Source: CAD feature listing. Evaluate the final solid. Frame: model axes, mm. A direction names the side the tool comes from. Give positions to 0.01 mm unless a question says otherwise; leave off trailing zeros. Loops run counter-clockwise (first coordinate to the right, second up) from the corner with the lowest first, then second, coordinate; pieces in that order, holes last. Notation, with made-up numbers: (9, 16.25) - (47, 16.25) arc R14 cw to (47, 20.25) - close; hole circle Ø5 at (89, 67). An arc over 180 degrees is marked (long way). Put each result on its own line as item: value.
```python
from build123d import *

# Parameters (mm, degrees)
F1_DEPTH  = 6.35
F0_W      = 7.9375
F0_H      = 7.9375
F2_DEPTH  = 12.7
F3_DEPTH  = 127
F5_DEPTH  = 50.8
F6_W      = 7.9502
F6_H      = 7.9502
F7_DEPTH  = 113.03
F8_W      = 44.45
F8_H      = 3.175
F9_DEPTH  = 6.35
F10_W     = 50.8
F10_H     = 3.175
F11_DEPTH = 3.175


with BuildPart() as f1:
    # F0 (on Top) → F1 (new body)
    with BuildSketch(Plane.XY):
        with BuildLine():
            ThreePointArc((-100.0125, -39.6875), (-96.292756, -48.667756), (-87.3125, -52.3875))
            Line((-87.3125, -52.3875), (87.3125, -52.3875))
            ThreePointArc((87.3125, -52.3875), (96.292756, -48.667756), (100.0125, -39.6875))
            Line((100.0125, -39.6875), (100.0125, 39.6875))
            ThreePointArc((100.0125, 39.6875), (96.292756, 48.667756), (87.3125, 52.3875))
            Line((87.3125, 52.3875), (-87.3125, 52.3875))
            ThreePointArc((-87.3125, 52.3875), (-96.292756, 48.667756), (-100.0125, 39.6875))
            Line((-100.0125, 39.6875), (-100.0125, -39.6875))
        make_face()
    extrude(amount=F1_DEPTH)

    # F0 (on Top) → F2 (join)
    with BuildSketch(Plane.XY):
        with BuildLine():
            Line((-100.0125, -39.6875), (-100.0125, -52.3875))
            Line((-100.0125, -52.3875), (-87.3125, -52.3875))
            ThreePointArc((-87.3125, -52.3875), (-96.292756, -48.667756), (-100.0125, -39.6875))
        make_face()
        Polygon((-107.95, 52.3875), (-107.95, -52.3875), (-100.0125, -52.3875), (-100.0125, -39.6875), (-100.0125, 39.6875), (-100.0125, 52.3875), align=None)
        Polygon((-100.0125, -52.3875), (-100.0125, -60.325), (100.0125, -60.325), (100.0125, -52.3875), (87.3125, -52.3875), (-87.3125, -52.3875), align=None)
        Polygon((-100.0125, 60.325), (-100.0125, 52.3875), (-87.3125, 52.3875), (87.3125, 52.3875), (100.0125, 52.3875), (100.0125, 60.325), align=None)
        with BuildLine():
            Line((-87.3125, 52.3875), (-100.0125, 52.3875))
            Line((-100.0125, 52.3875), (-100.0125, 39.6875))
            ThreePointArc((-100.0125, 39.6875), (-96.292756, 48.667756), (-87.3125, 52.3875))
        make_face()
        with BuildLine():
            ThreePointArc((87.3125, 52.3875), (96.292756, 48.667756), (100.0125, 39.6875))
            Line((100.0125, 39.6875), (100.0125, 52.3875))
            Line((100.0125, 52.3875), (87.3125, 52.3875))
        make_face()
        Polygon((100.0125, -39.6875), (100.0125, -52.3875), (107.95, -52.3875), (107.95, 52.3875), (100.0125, 52.3875), (100.0125, 39.6875), align=None)
        with BuildLine():
            Line((87.3125, -52.3875), (100.0125, -52.3875))
            Line((100.0125, -52.3875), (100.0125, -39.6875))
            ThreePointArc((100.0125, -39.6875), (96.292756, -48.667756), (87.3125, -52.3875))
        make_face()
        with Locations((103.98125, -56.35625)):
            Rectangle(F0_W, F0_H)
        with Locations((103.98125, 56.35625)):
            Rectangle(F0_W, F0_H)
        with Locations((-103.98125, 56.35625)):
            Rectangle(F0_W, F0_H)
        with Locations((-103.98125, -56.35625)):
            Rectangle(F0_W, F0_H)
    extrude(amount=F2_DEPTH)

    # F0 (on Top) → F3 (join)
    with BuildSketch(Plane.XY):
        with Locations((-103.98125, -56.35625)):
            Rectangle(F0_W, F0_H)
        with Locations((-103.98125, 56.35625)):
            Rectangle(F0_W, F0_H)
        with Locations((103.98125, 56.35625)):
            Rectangle(F0_W, F0_H)
        with Locations((103.98125, -56.35625)):
            Rectangle(F0_W, F0_H)
    extrude(amount=-F3_DEPTH)

    # F4 (on face) → F5 (join)
    with BuildSketch(Plane.XY.offset(12.7)):
        with BuildLine():
            ThreePointArc((0, 60.325), (-3.96875, 56.35625), (0, 52.3875))
            Line((0, 52.3875), (0, 60.325))
        make_face()
        with BuildLine():
            ThreePointArc((0, -52.3875), (-3.96875, -56.35625), (0, -60.325))
            Line((0, -60.325), (0, -52.3875))
        make_face()
        with BuildLine():
            Line((0, -52.3875), (0, -60.325))
            ThreePointArc((0, -60.325), (2.80633, -59.16258), (3.96875, -56.35625))
            ThreePointArc((3.96875, -56.35625), (2.80633, -53.54992), (0, -52.3875))
        make_face()
        with BuildLine():
            Line((-3.9751, -60.325), (0, -60.325))
            ThreePointArc((0, -60.325), (-3.96875, -56.35625), (0, -52.3875))
            Line((0, -52.3875), (-3.9751, -52.3875))
            Line((-3.9751, -52.3875), (-3.9751, -60.325))
        make_face()
        with BuildLine():
            ThreePointArc((3.96875, -56.35625), (2.80633, -59.16258), (0, -60.325))
            Line((0, -60.325), (3.9751, -60.325))
            Line((3.9751, -60.325), (3.9751, -52.3875))
            Line((3.9751, -52.3875), (0, -52.3875))
            ThreePointArc((0, -52.3875), (2.80633, -53.54992), (3.96875, -56.35625))
        make_face()
        with BuildLine():
            ThreePointArc((3.96875, 56.35625), (2.80633, 53.54992), (0, 52.3875))
            Line((0, 52.3875), (3.9751, 52.3875))
            Line((3.9751, 52.3875), (3.9751, 60.325))
            Line((3.9751, 60.325), (0, 60.325))
            ThreePointArc((0, 60.325), (2.80633, 59.16258), (3.96875, 56.35625))
        make_face()
        with BuildLine():
            Line((0, 60.325), (0, 52.3875))
            ThreePointArc((0, 52.3875), (2.80633, 53.54992), (3.96875, 56.35625))
            ThreePointArc((3.96875, 56.35625), (2.80633, 59.16258), (0, 60.325))
        make_face()
        with BuildLine():
            Line((-3.9751, 52.3875), (0, 52.3875))
            ThreePointArc((0, 52.3875), (-3.96875, 56.35625), (0, 60.325))
            Line((0, 60.325), (-3.9751, 60.325))
            Line((-3.9751, 60.325), (-3.9751, 52.3875))
        make_face()
    extrude(amount=F5_DEPTH)

    # F6 (on face) → F7 (join)
    with BuildSketch(Plane.XZ.offset(-52.3875)):
        with Locations((0, 59.5249)):
            Rectangle(F6_W, F6_H)
    extrude(amount=F7_DEPTH)

    # F8 (on face) → F9 (cut)
    with BuildSketch(Plane.YZ.offset(-100.0125)):
        with Locations((-0.538783, 7.9375)):
            Rectangle(F8_W, F8_H)
    extrude(amount=-F9_DEPTH, mode=Mode.SUBTRACT)

    # F10 (on face) → F11 (cut)
    with BuildSketch(Plane(origin=(100.0125, 0, 0), x_dir=(0, -1, 0), z_dir=(-1, 0, 0))):
        with Locations((0.075357, 7.9375)):
            Rectangle(F10_W, F10_H)
    extrude(amount=-F11_DEPTH, mode=Mode.SUBTRACT)


solid = f1.part
```
1) Section query B-B, the plane z = -107. State how many separate pieces and enclosed holes the cut face has, plus the area to 3 significant figures.
Check result:
separate pieces: 4
enclosed holes: 0
area: 252 mm²
2) Section query A-A, the plane y = 37. Output: boundary loops of the cut face in (x, z), plus the area to 3 significant figures.
Check result:
outline: (-107.95, 0) - (107.95, 0) - (107.95, 12.7) - (100.01, 12.7) - (100.01, 6.35) - (-100.01, 6.35) - (-100.01, 12.7) - (-107.95, 12.7) - close; (-3.98, 55.55) - (3.98, 55.55) - (3.98, 63.5) - (-3.98, 63.5) - close
area: 1,530 mm²
3) Mould query, pull axis Y, two halves, no side actions, for faces 1 (the flat face through (0, 1, 63.5)), 2 (the flat face through (0, 52.388, 14)), 3 (the flat face through (-1, -60.325, 5)). Classes: pulls with the +Y half, pulls with the -Y half, needs draft (parallel to the pull), parting line crosses it, or undercut.
Check result:
face 1: needs draft
face 2: undercut
face 3: pulls with the -Y half
4) Material intervals for line 1 along Y through (x, z) = (63, 11) (1 decimal); line 2 along X through (y, z) = (55.5, -88.5); line 3 along Z through (x, y) = (-78.5, 28.5), sorted ascending. Write a range as [from, to].
Check result:
line 1: [-60.3, -52.4], [52.4, 60.3]
line 2: [-107.95, -100.01], [100.01, 107.95]
line 3: [0, 6.35]
5) Section query C-C, the plane z = 26. Output: boundary loops of the cut face in (x, y) (1 decimal).
Check result:
outline: (-4, -60.3) - (4, -60.3) - (4, -52.4) - (-4, -52.4) - close; (-4, 52.4) - (4, 52.4) - (4, 60.3) - (-4, 60.3) - close
6) Pin query (flat end, axial travel): P1, Ø3, axis at x = 55.5, z = 9.5, coming from the -Y side (3 decimals); P2, Ø10, axis at x = -84.5, z = -3, coming from the +Y side (3 decimals); P3, Ø1.6, axis at x = 101.5, y = -11, coming from the -Z side; P4, Ø12, axis at x = 72, y = -44, coming from the +Z side. Return the tip coordinate at first contact, or that it passes through.
Check result:
P1: y = -60.325
P2: y = 60.325
P3: z = 0
P4: z = 6.35
7) Access query for faces 4 (the cylindrical face through (96.19, 48.77, 9.48)), 5 (the flat face through (0, -52.388, 14)), 6 (the flat face through (-102, 0, 12.7)), 7 (the flat face through (100.012, 56, -63)), 8 (the flat face through (3.975, 0, 57)). Directions: +Z, -Z, +X, -X, +Y, -Y. A direction counts if a zero-diameter tool reaches every point of the face in a straight line with its end or side. Return the directions, or none.
Check result:
face 4: +Z
face 5: none
face 6: +Z, -X, +Y, -Y
face 7: -Z, +Y, -Y
face 8: +Z, +X, +Y, -Y
